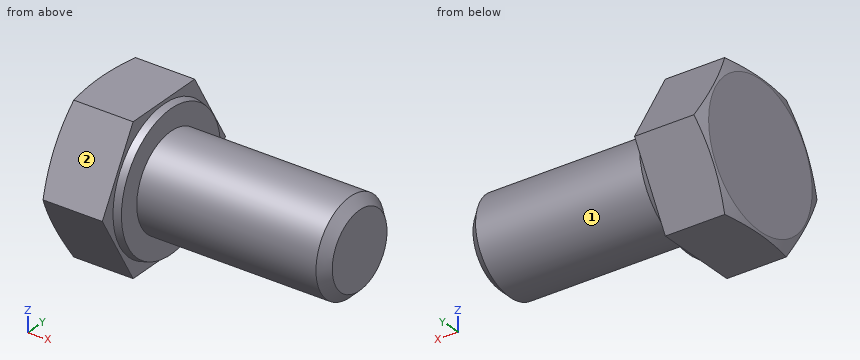
```python
from build123d import *

# Parameters (mm, degrees)
SKETCH_2_OUTSIDE_W  = 22.38
SKETCH_2_OUTSIDE_H  = 22.38
CUT_EXTRUDE_1_DEPTH = 25.281571201
CHAMFER_1_SIZE      = 0.8


with BuildPart() as part:
    # Эскиз1 → Повернуть1 (revolve)
    with BuildSketch(Plane.XY, mode=Mode.PRIVATE) as revolve_1_sk:
        Polygon((-5.45, 0), (-5.45, 7.19), (0, 7.19), (0, 5.948974596), (0.6, 5.788205081), (0.6, 4), (16.6, 4), (16.6, 0), align=None)
    revolve(revolve_1_sk.sketch.rotate(Axis((-1000, 0, 0), (1, 0, 0)), 90), axis=Axis((-1000, 0, 0), (1, 0, 0)))

    # Эскиз2 outside → Вырез-Вытянуть1 (cut, through all)
    with BuildSketch(Plane.ZY.offset(5.45)):
        Rectangle(SKETCH_2_OUTSIDE_W, SKETCH_2_OUTSIDE_H)
        Polygon((0, -7.19), (6.226722653, -3.595), (6.226722653, 3.595), (0, 7.19), (-6.226722653, 3.595), (-6.226722653, -3.595), align=None, mode=Mode.SUBTRACT)
    extrude(amount=-CUT_EXTRUDE_1_DEPTH, mode=Mode.SUBTRACT)

    # Эскиз4 → Вырез-Повернуть1 (revolve, cut)
    with BuildSketch(Plane.XY, mode=Mode.PRIVATE) as cut_revolve_1_sk:
        Polygon((-5.45, 6.04675), (-5.03389103, 7.19), (-5.45, 7.19), align=None)
    revolve(cut_revolve_1_sk.sketch.rotate(Axis((-1000, 0, 0), (1, 0, 0)), 299.999999983), axis=Axis((-1000, 0, 0), (1, 0, 0)), mode=Mode.SUBTRACT)

    # Фаска1
    chamfer_1_edges = [part.edges().sort_by_distance(p)[0] for p in [
        (16.6, 0, -4),
    ]]
    chamfer(chamfer_1_edges, length=CHAMFER_1_SIZE)


solid = part.part
```
The listing builds one solid part. Answer for the finished solid, in the listing's coordinates (mm). Face numbers are marked on the shaded views. A direction names the side the tool comes from. Give positions to 0.01 mm unless a question says otherwise; leave off trailing zeros. Order: outer loops, then holes, each group sorted by start corner. A loop starts at its lowest first (then second) coordinate and runs counter-clockwise, first axis right, second up. Notation, with made-up numbers: (87.5, 35.5) - (121.5, 35.5) arc R27 cw to (121.5, 66.5) - close; hole circle Ø11 at (-0.5, 86). An arc over 180 degrees is marked (long way). Answer in a Markdown table with one row per item. Add a question column.
Q1. Given P1, Ø6, axis at y = -1, z = 4, coming from the +X side; P2, Ø2, axis at x = 4.5, z = -1, coming from the -Y side; P3, Ø1.5, axis at x = 10.5, z = -3.5, coming from the +Y side; P4, Ø3, axis at x = 3, y = 2.5, coming from the +Z side, each flat-ended and moving along its own axis, determine where each tip first touches the part or whether it passes through.
Q2. Find the intervals of material crossed by line 1 along X through (y, z) = (4.5, -1); line 2 along Y through (x, z) = (7, -1.75); line 3 along Y through (x, z) = (3.25, 0), in increasing order. Write a range as [from, to].
Q3. The part is cut by section B-B (x = 1.5). Determine the outline of the cut face in (y, z).
Q4. Which of the six approach directions +Z, -Z, +X, -X, +Y, -Y give full straight-line access (tool end or side, diameter ignored) to the marked faces 1 and 2?
Q5. The part is cut by section A-A (y = 0). Determine the outline of the cut face in (x, z), then the cut area to 3 significant figures.
Determined:
| question | item | result |
|---|---|---|
| 1 | P1 | stops at x = 16.6 |
| 1 | P2 | stops at y = -4 |
| 1 | P3 | stops at y = 2.9 |
| 1 | P4 | stops at z = 3.87 |
| 2 | line 1 | x = [-5.45, 0.6] |
| 2 | line 2 | y = [-3.6, 3.6] |
| 2 | line 3 | y = [-4, 4] |
| 3 | outline | circle Ø8 at (0, 0) |
| 4 | face 1 | +X |
| 4 | face 2 | +Z, +X, -X, -Y |
| 5 | outline | (-5.45, -6.05) - (-5.38, -6.23) - (0, -6.23) - (0, -5.95) - (0.6, -5.79) - (0.6, -4) - (15.8, -4) - (16.6, -3.2) - (16.6, 3.2) - (15.8, 4) - (0.6, 4) - (0.6, 5.79) - (0, 5.95) - (0, 6.23) - (-5.38, 6.23) - (-5.45, 6.05) - close |
| 5 | area | 202 mm² |
